Work out the finished part from the listing and answer in its coordinate system (mm). Face numbers are marked on the shaded views. A direction names the side the tool comes from. Coordinates: 2 decimals unless noted, no trailing zeros. Order: outer loops, then holes, each group sorted by start corner. A loop starts at its lowest first (then second) coordinate and runs counter-clockwise, first axis right, second up. Notation, with made-up numbers: M 87,-35 L 103,-35 A29 cw 103,-10 Z; hole C 76.5,-20 d7. An arc over 180 degrees is marked long. Use a Markdown table: item, result. Add a question column.
from build123d import *

# Parameters (mm, degrees)
SKETCH4_OUTSIDE_W  = 22.004
SKETCH4_OUTSIDE_H  = 22.004
CUT_EXTRUDE1_DEPTH = 40.845535091


with BuildPart() as part:
    # Sketch3 → Revolve1 (revolve)
    with BuildSketch(Plane(origin=(0, 0, 0), x_dir=(0, 0, -1), z_dir=(1, 0, 0)), mode=Mode.PRIVATE) as revolve1_sk:
        Polygon((-19.5, 0), (-19.5, 4.8), (-18.937947959, 5.773502692), (-15.82, 5.773502692), (-15.82, 4.8), (-15.5, 4.8), (-15.5, 3), (18.8, 3), (19.5, 2.3), (19.5, 0), align=None)
    revolve(revolve1_sk.sketch.rotate(Axis((0, 0, 19.5), (0, 0, -1)), 90), axis=Axis((0, 0, 19.5), (0, 0, -1)))

    # Sketch4 outside → Cut-Extrude1 (cut, through all)
    with BuildSketch(Plane.XY.offset(19.5)):
        Rectangle(SKETCH4_OUTSIDE_W, SKETCH4_OUTSIDE_H)
        Polygon((5, 2.886751346), (0, 5.773502692), (-5, 2.886751346), (-5, -2.886751346), (0, -5.773502692), (5, -2.886751346), align=None, mode=Mode.SUBTRACT)
    extrude(amount=-CUT_EXTRUDE1_DEPTH, mode=Mode.SUBTRACT)


solid = part.part
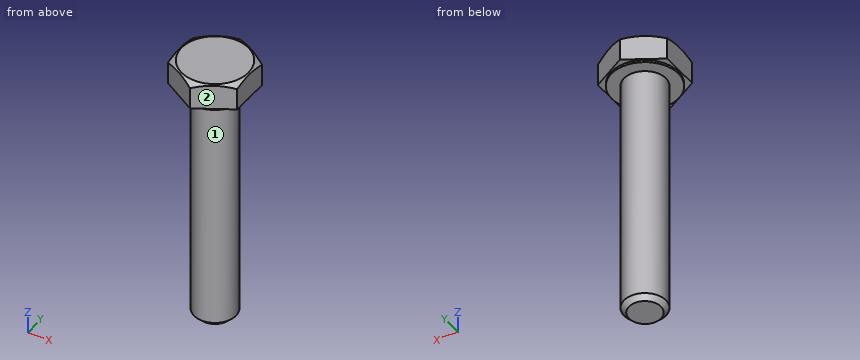
(1) A cutting plane is placed at B-B on z = 7. Write down the section's boundary in (x, y).
(2) Straight lines are drawn through the part: line 1 (Z direction, x = -3.25, y = 2); line 2 (Y direction, x = 2, z = -14.5); line 3 (X direction, y = -1.75, z = -8). For each, find the intervals that lie inside material, in ascending order.
(3) Given P1, Ø5, axis at y = 0.5, z = -8, coming from the +X side; P2, Ø3, axis at y = 0, z = 9, coming from the -X side; P3, Ø4, axis at x = 0.5, z = -13.5, coming from the -Y side, each flat-ended and moving along its own axis, determine where each tip first touches the part or whether it passes through.
(4) Which of the six approach directions +Z, -Z, +X, -X, +Y, -Y give full straight-line access (tool end or side, diameter ignored) to the marked faces 1 and 2?
(5) A cutting plane is placed at A-A on y = 0. Write down the section's boundary in (x, z), plus the area to 3 significant figures.
From the geometry:
| question | item | result |
|---|---|---|
| 1 | outline | C 0,0 d6 |
| 2 | line 1 | z = 15.5 to 19.5 |
| 2 | line 2 | y = -2.24 to 2.24 |
| 2 | line 3 | x = -2.44 to 2.44 |
| 3 | P1 | stops at x = 3 |
| 3 | P2 | stops at x = -3 |
| 3 | P3 | stops at y = -3 |
| 4 | face 1 | -Z |
| 4 | face 2 | +Z, -Z, +X, -Y |
| 5 | outline | M -5,15.82 L -4.8,15.82 L -4.8,15.5 L -3,15.5 L -3,-18.8 L -2.3,-19.5 L 2.3,-19.5 L 3,-18.8 L 3,15.5 L 4.8,15.5 L 4.8,15.82 L 5,15.82 L 5,19.38 L 4.8,19.5 L -4.8,19.5 L -5,19.38 Z |
| 5 | area | 249 mm2 |
